Model file for the job. Use its own axes, mm. Give positions to 0.01 mm unless a question says otherwise; leave off trailing zeros. Order: outer loops, then holes, each group sorted by start corner. A loop starts at its lowest first (then second) coordinate and runs counter-clockwise, first axis right, second up. Notation, with made-up numbers: (75.25, 62.5) - (89.25, 62.5) arc R20 cw to (89.25, 99.5) - close; hole circle Ø3 at (42, 48.25). An arc over 180 degrees is marked (long way). Return JSON: item names as keys, results as strings. Group by question number.
from build123d import *

# Parameters (mm, degrees)
SKETCH1_R               = 30
SKETCH1_R_2             = 22.5
BOSS_EXTRUDE2_DEPTH     = 145
CROQUIS1_R              = 5.5
CROQUIS1_R_2            = 3
SALIENTE_EXTRUIR1_DEPTH = 145
MATRIZC1_COUNT          = 4


with BuildPart() as part:
    # Sketch1 → Boss-Extrude2 (new body)
    with BuildSketch(Plane.XY):
        Circle(SKETCH1_R)
        Circle(SKETCH1_R_2, mode=Mode.SUBTRACT)
    extrude(amount=BOSS_EXTRUDE2_DEPTH)

    # Croquis1 → Saliente-Extruir1 (add)
    with BuildSketch(Plane.XY):
        with Locations((-33, 0)):
            Circle(CROQUIS1_R)
        with Locations((-33, 0)):
            Circle(CROQUIS1_R_2, mode=Mode.SUBTRACT)
    saliente_extruir1 = extrude(amount=SALIENTE_EXTRUIR1_DEPTH)

    # MatrizC1: Saliente-Extruir1 ×4 about axis
    matrizc1_axis = Axis((0, 0, 0), (0, 0, 1))
    for i in range(1, MATRIZC1_COUNT):
        add(saliente_extruir1.rotate(matrizc1_axis, i * 360 / MATRIZC1_COUNT))


solid = part.part
(1) Drill centre lines: L1, parallel to X at y = 33, z = 106; L2, parallel to X at y = -18, z = 19.5. Where is each one in solid material? Low to high.
(2) Pull direction X, two halves, no side cores. Call faces 1 (the face through (0, 36, 71)), 2 (the face through (20, 11, 145)): released by +X, released by -X, zero draft, split by the parting line, or undercut.
(3) Slice it at A-A (x = -33). Give the cut face in (y, z), and give its area (3 significant figures).
(4) Slice it at C-C (z = 62). Give the cut face in (x, y).
(5) Drop flat-ended pins along their axis: pin 1 Ø10 at (y, z) = (20, 26) entering from +X; pin 2 Ø2 at (x, z) = (-0.5, 104.5) entering from +Y; pin 3 Ø12 at (y, z) = (16, 69) entering from -X; pin 4 Ø1 at (y, z) = (26, 65.5) entering from +X. Give the stop position or say it passes through.
(6) Slice it at B-B (y = 0). Give the cut face in (x, z), and give its area (3 significant figures).
Result set:
{
 "1": {"L1": "x = -5.5 to -3, 3 to 5.5", "L2": "x = -24 to -13.5, 13.5 to 24"},
 "2": {"face 1": "undercut", "face 2": "zero draft"},
 "3": {"outline": "(-5.5, 0) - (-3, 0) - (-3, 145) - (-5.5, 145) - close; (3, 0) - (5.5, 0) - (5.5, 145) - (3, 145) - close", "area": "725 mm²"},
 "4": {"outline": "(-29.68, -4.38) arc R30 ccw to (-4.38, -29.68) arc R5.5 ccw (long way) to (4.38, -29.68) arc R30 ccw to (29.68, -4.38) arc R5.5 ccw (long way) to (29.68, 4.38) arc R30 ccw to (4.38, 29.68) arc R5.5 ccw (long way) to (-4.38, 29.68) arc R30 ccw to (-29.68, 4.38) arc R5.5 ccw (long way) to start; hole circle Ø6 at (-33, 0); hole circle Ø45 at (0, 0); hole circle Ø6 at (0, -33); hole circle Ø6 at (0, 33); hole circle Ø6 at (33, 0)"},
 "5": {"pin 1": "stops at x = 25.98", "pin 2": "stops at y = 38.5", "pin 3": "stops at x = -28.28", "pin 4": "stops at x = 15.8"},
 "6": {"outline": "(-38.5, 0) - (-36, 0) - (-36, 145) - (-38.5, 145) - close; (-30, 0) - (-22.5, 0) - (-22.5, 145) - (-30, 145) - close; (22.5, 0) - (30, 0) - (30, 145) - (22.5, 145) - close; (36, 0) - (38.5, 0) - (38.5, 145) - (36, 145) - close", "area": "2,900 mm²"}
}
